Verification items for the finished model (mm, model axes). Face numbers are marked on the shaded views. Give positions to 0.01 mm unless a question says otherwise; leave off trailing zeros. Order: outer loops, then holes, each group sorted by start corner. A loop starts at its lowest first (then second) coordinate and runs counter-clockwise, first axis right, second up. Notation, with made-up numbers: (28, 20.25) - (81, 20.25) arc R16 ccw to (81, 45.25) - close; hole circle Ø7 at (-9, 1.5). An arc over 180 degrees is marked (long way). Answer as a JSON object with one key per item and string values. Group by question number.
(1) Section check C-C (x = -18). Record the boundary of the cut face in (y, z).
(2) Mould release check, pull along Z, two halves, no side actions. Record for the marked faces 1 and 2: +Z half, -Z half, draft (parallel to the pull), parting line (faces both ways), or undercut.
(3) Section check A-A (z = -37.5). Record the boundary of the cut face in (x, y).
(4) Section check B-B (y = 1.5). Record the boundary of the cut face in (x, z), then the cut area to 3 significant figures.
(5) Depth check by flat-ended pin: pin 1 Ø12 at (x, z) = (4, -12) entering from -Y; pin 2 Ø3.5 at (x, y) = (-1.5, 6) entering from -Z; pin 3 Ø1.2 at (y, z) = (6.5, -52) entering from -X. Enter the tip coordinate at first touch or a pass-through.
(6) Thickness scan on line 1 (X direction, y = 1.25, z = 0); line 2 (Z direction, x = -40.5, y = 0.75); line 3 (X direction, y = 6.75, z = -56.5). Record the ranges inside material, lowest first.
(7) Section check D-D (z = -13.5). Record the boundary of the cut face in (x, y).
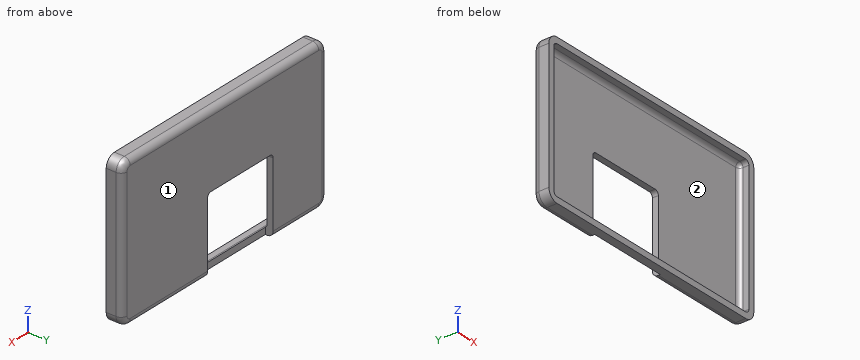
Autodesk Inventor part; units mm, degrees
ref_plane "YZ Plane" through (0, 0, 0) normal (1, 0, 0) x (0, 1, 0)
ref_plane "XZ Plane" through (0, 0, 0) normal (0, 1, 0) x (-1, 0, 0)
ref_plane "XY Plane" through (0, 0, 0) normal (0, 0, 1) x (1, 0, 0)
sketch "Sketch1" plane through (0, 0, 0) normal (0, 1, 0) x (-1, 0, 0)
  line L0 (57.5, -65) -> (-57.5, -65)
  line L1 (-62.5, -60) -> (-62.5, 5)
  line L2 (-57.5, 10) -> (57.5, 10)
  line L3 (62.5, 5) -> (62.5, -60)
  arc A0 (-57.5, 10) -> (-62.5, 5) centre (-57.5, 5) ccw
  arc A1 (62.5, 5) -> (57.5, 10) centre (57.5, 5) ccw
  arc A2 (57.5, -65) -> (62.5, -60) centre (57.5, -60) ccw
  arc A3 (-62.5, -60) -> (-57.5, -65) centre (-57.5, -60) ccw
  line L4 (0, 10) -> (0, -20.4446) construction
  point P0 (0, 0)
  point P1 (62.5, -65)
  point P2 (-62.5, 10)
  point P3 (62.5, 10)
  dimension "d0" = 125
  dimension "d4" = 75
  dimension "d5" = 5
  dimension "d9" = 10
extrude "Extrusion1" add sketch "Sketch1" along normal blind 8
fillet "Fillet1" radius 3 8 edges at (-61.0355, 8, 8.5355) (0, 8, 10) (61.0355, 8, 8.5355) (62.5, 8, -27.5) (61.0355, 8, -63.5355) (0, 8, -65) (-61.0355, 8, -63.5355) (-62.5, 8, -27.5)
sketch "Sketch2" plane through (0, 0, 0) normal (0, -1, 0) x (1, 0, 0)
  line L0 (62.5, 5) -> (62.5, -60)
  arc A0 (62.5, 5) -> (57.5, 10) centre (57.5, 5) ccw
  line L1 (-57.5, 10) -> (57.5, 10)
  arc A1 (-57.5, 10) -> (-62.5, 5) centre (-57.5, 5) ccw
  line L2 (-62.5, -60) -> (-62.5, 5)
  arc A2 (-62.5, -60) -> (-57.5, -65) centre (-57.5, -60) ccw
  line L3 (57.5, -65) -> (-57.5, -65)
  arc A3 (57.5, -65) -> (62.5, -60) centre (57.5, -60) ccw
  arc A4 (59.5, 5) -> (57.5, 7) centre (57.5, 5) ccw
  line L4 (59.5, 5) -> (59.5, -60)
  arc A5 (57.5, -62) -> (59.5, -60) centre (57.5, -60) ccw
  line L5 (57.5, -62) -> (-57.5, -62)
  arc A6 (-59.5, -60) -> (-57.5, -62) centre (-57.5, -60) ccw
  line L6 (-59.5, -60) -> (-59.5, 5)
  arc A7 (-57.5, 7) -> (-59.5, 5) centre (-57.5, 5) ccw
  line L7 (-57.5, 7) -> (57.5, 7)
  point P0 (0, 0)
  dimension "d10" = 3
extrude "Extrusion2" cut sketch "Sketch2" against normal blind 5 contours L4 A5 L5 A6 L6 A7 L7 A4
fillet "Fillet2" radius 2 8 edges at (-58.9142, 5, -61.4142) (-59.5, 5, -27.5) (-58.9142, 5, 6.4142) (0, 5, 7) (58.9142, 5, 6.4142) (59.5, 5, -27.5) (58.9142, 5, -61.4142) (0, 5, -62)
sketch "Sketch3" plane through (0, 8, 0) normal (0, 1, 0) x (1, 0, 0)
  line L0 (-57.5, 62) -> (57.5, 62)
  line L1 (-27.7, 67) -> (8.3, 67)
  line L2 (10.3, 65) -> (10.3, 29)
  line L3 (8.3, 27) -> (-27.7, 27)
  line L4 (-29.7, 29) -> (-29.7, 65)
  arc A0 (-27.7, 67) -> (-29.7, 65) centre (-27.7, 65) ccw
  arc A1 (10.3, 65) -> (8.3, 67) centre (8.3, 65) ccw
  arc A2 (8.3, 27) -> (10.3, 29) centre (8.3, 29) ccw
  arc A3 (-29.7, 29) -> (-27.7, 27) centre (-27.7, 29) ccw
  line L5 (62.5, -5) -> (62.5, 60)
  line L6 (-62.5, 60) -> (-62.5, -5)
  point P0 (0, 0)
  point P1 (10.3, 27)
  point P2 (10.3, 67)
  point P3 (-29.7, 27)
  point P4 (-9.7, 67)
  dimension "d14" = 40
  dimension "d15" = 40
  dimension "d16" = 2
  dimension "d17" = 5
  dimension "d21" = 52.8
extrude "Extrusion3" cut sketch "Sketch3" against normal blind 4
properties part number "Beta_V2_Top01"
Solutions:
{
 "1": {"outline": "(0, -65) - (4, -65) - (4, -61.73) arc R2 cw to (3, -62) - (0, -62) - close; (0, 7) - (3, 7) arc R2 cw to (5, 5) - (5, -27) - (8, -27) - (8, 7) arc R3 ccw to (5, 10) - (0, 10) - close"},
 "2": {"face 1": "draft", "face 2": "undercut"},
 "3": {"outline": "(-62.5, 0) - (-59.5, 0) - (-59.5, 3) arc R2 cw to (-57.5, 5) - (-29.7, 5) - (-29.7, 8) - (-59.5, 8) arc R3 ccw to (-62.5, 5) - close; (10.3, 5) - (57.5, 5) arc R2 cw to (59.5, 3) - (59.5, 0) - (62.5, 0) - (62.5, 5) arc R3 ccw to (59.5, 8) - (10.3, 8) - close"},
 "4": {"outline": "(-62.5, -60) arc R5 ccw to (-57.5, -65) - (57.5, -65) arc R5 ccw to (62.5, -60) - (62.5, 5) arc R5 ccw to (57.5, 10) - (-57.5, 10) arc R5 ccw to (-62.5, 5) - close; hole (-59.5, -60) arc R2 ccw to (-57.5, -62) - (57.5, -62) arc R2 ccw to (59.5, -60) - (59.5, 5) arc R2 ccw to (57.5, 7) - (-57.5, 7) arc R2 ccw to (-59.5, 5) - close", "area": "1,150 mm2"},
 "5": {"pin 1": "stops at y = 5", "pin 2": "stops at z = -27", "pin 3": "stops at x = -62.36"},
 "6": {"line 1": "x = -62.5 to -59.5, 59.5 to 62.5", "line 2": "z = -65 to -62, 7 to 10", "line 3": "x = -61.94 to -29.7, 10.3 to 61.94"},
 "7": {"outline": "(-62.5, 0) - (-59.5, 0) - (-59.5, 3) arc R2 cw to (-57.5, 5) - (57.5, 5) arc R2 cw to (59.5, 3) - (59.5, 0) - (62.5, 0) - (62.5, 5) arc R3 ccw to (59.5, 8) - (-59.5, 8) arc R3 ccw to (-62.5, 5) - close"}
}
